The model under review builds one solid part; all positions refer to its coordinate system, in mm. Round coordinates to 2 decimals unless told otherwise and drop trailing zeros. Loops run counter-clockwise (first coordinate to the right, second up) from the corner with the lowest first, then second, coordinate; pieces in that order, holes last. Notation, with made-up numbers: M 61,-17.5 L 103,-17.5 A13 ccw 103,2.5 Z; hole C 13.5,44.5 d2. An arc over 180 degrees is marked long. Return JSON: item names as keys, results as strings. Group by question number.
Q1. Consider section A-A (z = 8.5). State the section outline as (x, y) points, and give its area (3 significant figures).
Q2. Draft analysis for pull direction Y (two halves, no side actions). For faces 1 (the face through (10.302, 16.228, 40.338)), 2 (the face through (10.302, -16.228, -40.338)), 3 (the face through (1.53, 2.75, 40.42)), state which applies: pulls with the +Y half, pulls with the -Y half, needs draft (parallel to the pull), parting line crosses it, or undercut.
Q3. Clearance check with a flat-ended pin moving along its axis: pin 1 Ø1.5 at (x, y) = (11.5, -14) entering from +Z. State where the tip first meets the part, or that it passes through.
Q4. To check wall thickness, follow line 1 along Y through (x, z) = (4.75, 28); line 2 along Y through (x, z) = (21.75, 31.5); line 3 along X through (y, z) = (-14, 15). State the ranges of each line that lie inside material, in increasing order.
Q5. Consider section B-B (x = 22.5). State the section outline as (y, z) points, and give its area (3 significant figures).
from build123d import *

# Parameters (mm, degrees)
F0_W     = 35.353254
F0_H     = 83.731398
F1_DEPTH = 25.4
F2_R     = 5.08


with BuildPart() as f1:
    # F0 (on Right) → F1 (new body)
    with BuildSketch(Plane.YZ):
        Rectangle(F0_W, F0_H)
    extrude(amount=F1_DEPTH)

    # F2
    f2_edges = [f1.edges().sort_by_distance(p)[0] for p in [
        (12.7, -17.676627, 41.865699),
        (25.4, 0, 41.865699),
        (12.7, 17.676627, 41.865699),
        (0, 0, 41.865699),
        (25.4, -17.676627, 0),
        (25.4, 17.676627, 0),
        (0, -17.676627, 0),
        (12.7, -17.676627, -41.865699),
        (25.4, 0, -41.865699),
    ]]
    fillet(f2_edges, radius=F2_R)


solid = f1.part
Values:
{
 "1": {"outline": "M 0,-12.6 A5.08 ccw 5.08,-17.68 L 20.32,-17.68 A5.08 ccw 25.4,-12.6 L 25.4,12.6 A5.08 ccw 20.32,17.68 L 0,17.68 Z", "area": "881 mm2"},
 "2": {"face 1": "pulls with the +Y half", "face 2": "pulls with the -Y half", "face 3": "needs draft"},
 "3": {"pin 1": "stops at z = 41.82"},
 "4": {"line 1": "y = -17.67 to 17.68", "line 2": "y = -17.47 to 17.47", "line 3": "x = 0.2 to 25.2"},
 "5": {"outline": "M -17.19,-36.79 A4.59 ccw -12.6,-41.37 L 17.19,-41.37 L 17.19,36.79 A4.59 ccw 12.6,41.37 L -12.6,41.37 A4.59 ccw -17.19,36.79 Z", "area": "2,830 mm2"}
}
